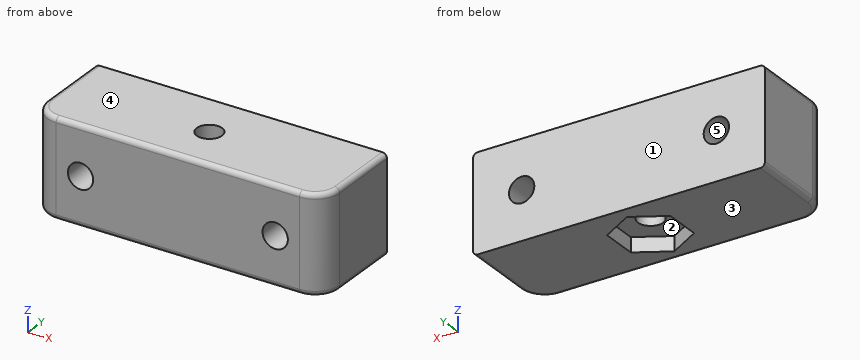
```python
from build123d import *

# Parameters (mm, degrees)
SKETCH1_R           = 2.6
BOSS_EXTRUDE1_DEPTH = 20
SKETCH2_R           = 2.6
CUT_EXTRUDE1_DEPTH  = 20
CUT_EXTRUDE2_DEPTH  = 3
FILLET1_R           = 1


with BuildPart() as part:
    # Sketch1 → Boss-Extrude1 (new body)
    with BuildSketch(Plane.XY):
        with BuildLine():
            Line((-30, 0), (30, 0))
            Line((30, 0), (30, -15))
            ThreePointArc((30, -15), (28.535533906, -18.535533906), (25, -20))
            Line((25, -20), (-25, -20))
            ThreePointArc((-25, -20), (-28.535533906, -18.535533906), (-30, -15))
            Line((-30, -15), (-30, 0))
        make_face()
        with Locations((0, -10)):
            Circle(SKETCH1_R, mode=Mode.SUBTRACT)
    extrude(amount=BOSS_EXTRUDE1_DEPTH)

    # Sketch2 → Cut-Extrude1 (cut)
    with BuildSketch(Plane(origin=(0, 0, 0), x_dir=(1, 0, 0), z_dir=(0, 1, 0))):
        with Locations((-20, -10)):
            Circle(SKETCH2_R)
        with Locations((20, -10)):
            Circle(SKETCH2_R)
    extrude(amount=-CUT_EXTRUDE1_DEPTH, mode=Mode.SUBTRACT)

    # Sketch3 → Cut-Extrude2 (cut)
    with BuildSketch(Plane(origin=(0, 0, 0), x_dir=(-1, 0, 0), z_dir=(0, 0, -1))):
        Polygon((0, -17.505553499), (6.5, -13.75277675), (6.5, -6.24722325), (0, -2.494446501), (-6.5, -6.24722325), (-6.5, -13.75277675), align=None)
    extrude(amount=-CUT_EXTRUDE2_DEPTH, mode=Mode.SUBTRACT)

    # Fillet1
    fillet1_edges = [part.edges().sort_by_distance(p)[0] for p in [
        (0, -20, 20),
        (28.535533906, -18.535533906, 20),
        (30, -7.5, 20),
        (-30, -7.5, 20),
        (30, -7.5, 0),
        (28.535533906, -18.535533906, 0),
        (-28.535533906, -18.535533906, 20),
        (0, -20, 0),
        (-28.535533906, -18.535533906, 0),
        (-30, -7.5, 0),
    ]]
    fillet(fillet1_edges, radius=FILLET1_R)


solid = part.part
```
Source: CAD feature listing. Evaluate the final solid. Frame: model axes, mm. Face numbers are marked on the shaded views. A direction names the side the tool comes from. Round coordinates to 2 decimals unless told otherwise and drop trailing zeros. Loops run counter-clockwise (first coordinate to the right, second up) from the corner with the lowest first, then second, coordinate; pieces in that order, holes last.
(1) Section query D-D (z = 3.75). Output: boundary loops of the cut face in (x, y).
From the geometry:
outline: (-30, -15) arc R5 ccw to (-25, -20) - (25, -20) arc R5 ccw to (30, -15) - (30, 0) - (-30, 0) - close; hole circle Ø5.2 at (0, -10)
(2) Section query C-C (x = 19). Output: boundary loops of the cut face in (y, z).
From the geometry:
outline: (-20, 1) arc R1 ccw to (-19, 0) - (0, 0) - (0, 7.6) - (-20, 7.6) - close; (-20, 12.4) - (0, 12.4) - (0, 20) - (-19, 20) arc R1 ccw to (-20, 19) - close
(3) Section query A-A (y = -9). Output: boundary loops of the cut face in (x, z).
From the geometry:
outline: (-30, 1) arc R1 ccw to (-29, 0) - (-6.5, 0) - (-6.5, 3) - (-2.4, 3) - (-2.4, 20) - (-29, 20) arc R1 ccw to (-30, 19) - close; (2.4, 3) - (6.5, 3) - (6.5, 0) - (29, 0) arc R1 ccw to (30, 1) - (30, 19) arc R1 ccw to (29, 20) - (2.4, 20) - close; hole circle Ø5.2 at (-20, 10); hole circle Ø5.2 at (20, 10)
(4) Pull-direction query (Z, two-part tool) for the marked faces 3, 4 and 5; classes: +Z half, -Z half, draft (parallel to the pull), parting line (faces both ways), or undercut.
From the geometry:
face 3: -Z half
face 4: +Z half
face 5: undercut
(5) Contact query for flat-ended pins moving along their axis: pin 1 Ø4 at (x, y) = (0, -10) entering from +Z; pin 2 Ø4 at (x, y) = (-2.5, -12) entering from -Z. Output: stop coordinate, or through.
From the geometry:
pin 1: passes through
pin 2: stops at z = 3
(6) Section query B-B (z = 11). Output: boundary loops of the cut face in (x, y), and give its area (3 significant figures).
From the geometry:
outline: (-30, -15) arc R5 ccw to (-25, -20) - (-22.4, -20) - (-22.4, 0) - (-30, 0) - close; (-17.6, -20) - (17.6, -20) - (17.6, 0) - (-17.6, 0) - close; (22.4, -20) - (25, -20) arc R5 ccw to (30, -15) - (30, 0) - (22.4, 0) - close; hole circle Ø5.2 at (0, -10)
area: 976 mm2
(7) Access query for the marked faces 1 and 2. Directions: +Z, -Z, +X, -X, +Y, -Y. A direction counts if a zero-diameter tool reaches every point of the face in a straight line with its end or side. Return the directions, or none.
From the geometry:
face 1: +Z, -Z, +X, -X, +Y
face 2: -Z
(8) Material intervals for probe 1 along X at (y, z) = (-4.25, 10); probe 2 along X at (y, z) = (-10.25, 8); probe 3 along X at (y, z) = (-10, 7), sorted ascending.
From the geometry:
probe 1: x = -30 to -22.6, -17.4 to 17.4, 22.6 to 30
probe 2: x = -30 to -21.66, -18.34 to -2.59, 2.59 to 18.34, 21.66 to 30
probe 3: x = -30 to -2.6, 2.6 to 30
